```python
from build123d import *

# Parameters (mm, degrees)
SKETCH1_W                      = 156.894022
SKETCH1_H                      = 71.14794
BOSS_EXTRUDE1_DEPTH            = 6.35
FILLET1_R                      = 3.175
CBORE_FOR_M3_SHCS1_D           = 3.6
CBORE_FOR_M3_SHCS1_CBORE_D     = 6.5
CBORE_FOR_M3_SHCS1_CBORE_DEPTH = 3
SHELL1_DEPTH                   = 3.175
SHELL1_2_DEPTH                 = 0.175
SKETCH8_W                      = 7.62
SKETCH8_H                      = 6.858
BOSS_EXTRUDE2_DEPTH            = 6.35
SKETCH9_R                      = 5.842
BOSS_EXTRUDE3_DEPTH            = 3.175
CUT_EXTRUDE2_START             = -1.5875
SKETCH10_R                     = 4.318
CUT_EXTRUDE2_DEPTH             = 2.794


# Read off the part's stored shape, not the designer's step: Shell1
with BuildPart() as part:
    # Sketch1 → Boss-Extrude1 (new body)
    with BuildSketch(Plane(origin=(0, 0, 0), x_dir=(1, 0, 0), z_dir=(0, 1, 0))):
        with Locations((78.447011, 35.57397)):
            Rectangle(SKETCH1_W, SKETCH1_H)
    extrude(amount=BOSS_EXTRUDE1_DEPTH)

    # Fillet1
    fillet1_edges = [part.edges().sort_by_distance(p)[0] for p in [
        (0, 3.175, -71.14794),
        (156.894022, 3.175, -71.14794),
        (156.894022, 3.175, 0),
        (0, 3.175, 0),
    ]]
    fillet(fillet1_edges, radius=FILLET1_R)

    # CBORE for M3 SHCS1 (through all)
    with Locations(Plane(origin=(0, 6.35, 0), x_dir=(1, 0, 0), z_dir=(0, 1, 0))):
        with Locations((3.96875, 67.17919), (31.75, 67.17919), (152.92524554, 67.17919), (3.96875, 3.96875), (104.48544, 3.96875), (152.92524554, 3.96875)):
            CounterBoreHole(CBORE_FOR_M3_SHCS1_D / 2, CBORE_FOR_M3_SHCS1_CBORE_D / 2, CBORE_FOR_M3_SHCS1_CBORE_DEPTH)

    # Shell1 outline → Shell1 (cut)
    with BuildSketch(Plane(origin=(0, 0, 0), x_dir=(1, 0, 0), z_dir=(0, 1, 0))):
        with BuildLine():
            Line((25.374218798, 67.97294), (10.344531202, 67.97294))
            ThreePointArc((10.344531202, 67.97294), (8.511911069, 62.636028931), (3.175, 60.803408798))
            Line((3.175, 60.803408798), (3.175, 10.344531202))
            ThreePointArc((3.175, 10.344531202), (8.511911069, 8.511911069), (10.344531202, 3.175))
            Line((10.344531202, 3.175), (98.109658798, 3.175))
            ThreePointArc((98.109658798, 3.175), (104.48544, 10.39375), (110.861221202, 3.175))
            Line((110.861221202, 3.175), (146.549464337, 3.175))
            ThreePointArc((146.549464337, 3.175), (148.382093898, 8.511920497), (153.719022, 10.344527908))
            Line((153.719022, 10.344527908), (153.719022, 60.803412092))
            ThreePointArc((153.719022, 60.803412092), (148.382093898, 62.636019503), (146.549464337, 67.97294))
            Line((146.549464337, 67.97294), (38.125781202, 67.97294))
            ThreePointArc((38.125781202, 67.97294), (31.75, 60.75419), (25.374218798, 67.97294))
        make_face()
    extrude(amount=SHELL1_DEPTH, mode=Mode.SUBTRACT)

    # Shell1 2 outline → Shell1 2 (cut)
    with BuildSketch(Plane(origin=(0, 0, 0), x_dir=(1, 0, 0), z_dir=(0, 1, 0))):
        with BuildLine():
            Line((10.344531202, 67.97294), (8.880021316, 67.97294))
            ThreePointArc((8.880021316, 67.97294), (7.486606236, 63.661333764), (3.175, 62.267918684))
            Line((3.175, 62.267918684), (3.175, 60.803408798))
            ThreePointArc((3.175, 60.803408798), (8.511911069, 62.636028931), (10.344531202, 67.97294))
        make_face()
        with BuildLine():
            Line((26.838728684, 67.97294), (25.374218798, 67.97294))
            ThreePointArc((25.374218798, 67.97294), (31.75, 60.75419), (38.125781202, 67.97294))
            Line((38.125781202, 67.97294), (36.661271316, 67.97294))
            ThreePointArc((36.661271316, 67.97294), (31.75, 62.20419), (26.838728684, 67.97294))
        make_face()
        with BuildLine():
            ThreePointArc((10.344531202, 3.175), (8.511911069, 8.511911069), (3.175, 10.344531202))
            Line((3.175, 10.344531202), (3.175, 8.880021316))
            ThreePointArc((3.175, 8.880021316), (7.486606236, 7.486606236), (8.880021316, 3.175))
            Line((8.880021316, 3.175), (10.344531202, 3.175))
        make_face()
        with BuildLine():
            Line((148.013974224, 67.97294), (146.549464337, 67.97294))
            ThreePointArc((146.549464337, 67.97294), (148.382093898, 62.636019503), (153.719022, 60.803412092))
            Line((153.719022, 60.803412092), (153.719022, 62.267922961))
            ThreePointArc((153.719022, 62.267922961), (149.40739878, 63.661324287), (148.013974224, 67.97294))
        make_face()
        with BuildLine():
            ThreePointArc((110.861221202, 3.175), (104.48544, 10.39375), (98.109658798, 3.175))
            Line((98.109658798, 3.175), (99.574168684, 3.175))
            ThreePointArc((99.574168684, 3.175), (104.48544, 8.94375), (109.396711316, 3.175))
            Line((109.396711316, 3.175), (110.861221202, 3.175))
        make_face()
        with BuildLine():
            Line((153.719022, 8.880017039), (153.719022, 10.344527908))
            ThreePointArc((153.719022, 10.344527908), (148.382093898, 8.511920497), (146.549464337, 3.175))
            Line((146.549464337, 3.175), (148.013974224, 3.175))
            ThreePointArc((148.013974224, 3.175), (149.40739878, 7.486615713), (153.719022, 8.880017039))
        make_face()
    extrude(amount=SHELL1_2_DEPTH, mode=Mode.SUBTRACT)

    # Sketch8 → Boss-Extrude2 (add)
    with BuildSketch(Plane.XZ.offset(-3.175)):
        with Locations((15.875, -11.684)):
            Rectangle(SKETCH8_W, SKETCH8_H)
        with Locations((15.875, -35.06597)):
            Rectangle(SKETCH8_W, SKETCH8_H)
        with Locations((15.875, -58.44794)):
            Rectangle(SKETCH8_W, SKETCH8_H)
        with Locations((129.89596777, -35.58794)):
            Rectangle(SKETCH8_W, SKETCH8_H)
    extrude(amount=BOSS_EXTRUDE2_DEPTH)

    # Sketch9 → Boss-Extrude3 (add)
    with BuildSketch(Plane.XZ.offset(-3.175)):
        with Locations((5.842, -23.374985)):
            Circle(SKETCH9_R)
        with Locations((5.842, -46.756955)):
            Circle(SKETCH9_R)
        with Locations((31.75, -5.842)):
            Circle(SKETCH9_R)
        with Locations((104.48544, -65.30594)):
            Circle(SKETCH9_R)
        with Locations((151.052022, -35.58794)):
            Circle(SKETCH9_R)
    extrude(amount=BOSS_EXTRUDE3_DEPTH)

    # Sketch10 → Cut-Extrude2 (cut)
    with BuildSketch(Plane(origin=(0, 6.35, 0), x_dir=(1, 0, 0), z_dir=(0, 1, 0)).offset(CUT_EXTRUDE2_START)):
        with Locations(Location((31.75, 5.842, 0), (0, 0, 270))):
            Circle(SKETCH10_R)
        with Locations(Location((5.842, 23.374985, 0), (0, 0, 270))):
            Circle(SKETCH10_R)
        with Locations(Location((5.842, 46.756955, 0), (0, 0, 270))):
            Circle(SKETCH10_R)
        with Locations(Location((104.48544, 65.30594, 0), (0, 0, 270))):
            Circle(SKETCH10_R)
        with Locations(Location((151.052022, 35.58794, 0), (0, 0, 270))):
            Circle(SKETCH10_R)
    extrude(amount=-CUT_EXTRUDE2_DEPTH, mode=Mode.SUBTRACT)


solid = part.part
```
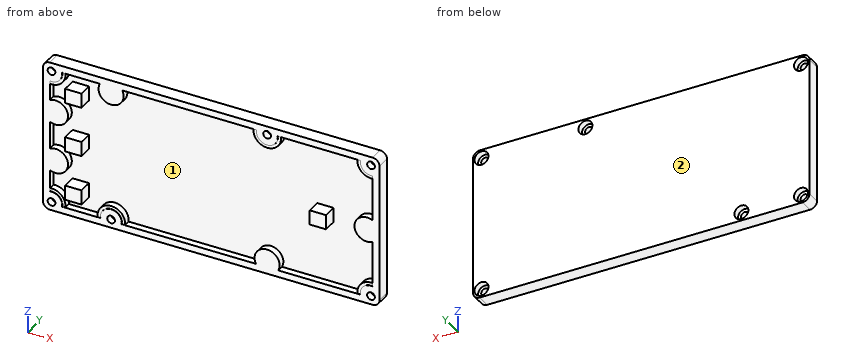
The model under review builds one solid part; all positions refer to its coordinate system, in mm. Face numbers are marked on the shaded views. Round coordinates to 2 decimals unless told otherwise and drop trailing zeros. Loops run counter-clockwise (first coordinate to the right, second up) from the corner with the lowest first, then second, coordinate; pieces in that order, holes last. Notation, with made-up numbers: (-2.75, -6.5) -> (1.25, -6.5) arc R28 cw to (1.25, 24.5) -> close; hole circle Ø5 at (47, 34.5). An arc over 180 degrees is marked (long way). Answer as a JSON object with one key per item and string values. Group by question number.
1) We need section A-A on x = 31.75. Give the number of separate pieces and of enclosed holes in the cut face, then the cut area to 3 significant figures.
2) Mouldability with a two-part tool opening along Z and no side actions: class the marked faces 1 and 2 as released by +Z, released by -Z, zero draft, split by the parting line, or undercut.
3) We need section C-C on x = 124. Write out the cut boundary in (y, z) (3 decimals), then the cut area to 3 significant figures.
4) For line 1 (X direction, y = 2, z = -13) (3 decimals); line 2 (Z direction, x = 15, y = 0.25) (3 decimals); line 3 (Z direction, x = 20.5, y = 0.5) (3 decimals), list the stretches that pass through material, from the lowest coordinate up. Write a range as [from, to].
5) For pin 1 Ø1.9 at (y, z) = (-1, -36.5) entering from -X (3 decimals); pin 2 Ø2.5 at (x, z) = (149.5, -36) entering from -Y; pin 3 Ø2 at (x, z) = (55, -64) entering from -Y (3 decimals); pin 4 Ø4 at (x, z) = (19.5, -8) entering from -Y (3 decimals), all flat-tipped, find the tip position at first contact; note any pin that passes through.
6) We need section B-B on x = 14. Write out the cut boundary in (y, z) (3 decimals), then the cut area to 3 significant figures.
Result set:
{
 "1": {"separate pieces": "2", "enclosed holes": "1", "area": "240 mm²"},
 "2": {"face 1": "undercut", "face 2": "zero draft"},
 "3": {"outline": "(0, -71.148) -> (6.35, -71.148) -> (6.35, 0) -> (0, 0) -> (0, -3.175) -> (3.175, -3.175) -> (3.175, -67.973) -> (0, -67.973) -> close", "area": "246 mm²"},
 "4": {"line 1": "[0, 3.175], [12.065, 19.685], [153.719, 156.894]", "line 2": "[-71.148, -67.973], [-61.877, -55.019], [-38.495, -31.637], [-15.113, -8.255], [-3.175, 0]", "line 3": "[-71.148, -67.973], [-3.175, 0]"},
 "5": {"pin 1": "x = 12.065", "pin 2": "y = 0", "pin 3": "y = 3.175", "pin 4": "y = -3.175"},
 "6": {"outline": "(-3.175, -61.877) -> (3.175, -61.877) -> (3.175, -67.973) -> (0, -67.973) -> (0, -71.148) -> (6.35, -71.148) -> (6.35, 0) -> (0, 0) -> (0, -3.175) -> (3.175, -3.175) -> (3.175, -8.255) -> (-3.175, -8.255) -> (-3.175, -15.113) -> (3.175, -15.113) -> (3.175, -31.637) -> (-3.175, -31.637) -> (-3.175, -38.495) -> (3.175, -38.495) -> (3.175, -55.019) -> (-3.175, -55.019) -> close", "area": "377 mm²"}
}
